Build history of the part. All positions in model axes, mm. A direction names the side the tool comes from. Give positions to 0.01 mm unless a question says otherwise; leave off trailing zeros. Write each loop counter-clockwise with the first axis right and the second up, starting at its lowest first coordinate (ties: lowest second). Pieces come first, ordered by that corner, then holes. Notation, with made-up numbers: (-7, 57) -> (19, 57) arc R5 ccw to (19, 64) -> close; hole circle Ø3 at (11, 8). An arc over 180 degrees is marked (long way). One line per question, with ' | ' between items. Start each with the question number.
(1) Tool access for faces 4 (the flat face through (-2.5, 0, -1)), 5 (the cylindrical face through (-1.43, 0.13, 0.45)), 6 (the flat face through (2.5, 0, -1)): list every direction of +Z, -Z, +X, -X, +Y, -Y with a clear straight run to the whole face (end or side of a thin tool).
(2) Pin check, flat tips, straight feed: P1, Ø0.6, axis at y = -2, z = -1, coming from the +X side; P2, Ø8, axis at x = 5, y = 5, coming from the -Z side; P3, Ø1, axis at y = 2.5, z = -1, coming from the -X side; P4, Ø7, axis at x = 6.5, y = 1.5, coming from the -Z side. Stop position of each tip, or through.
(3) Band-saw the part on C-C, the plane z = 2.5. Give the cut face in (x, y).
(4) Pull direction X, two halves, no side cores. Call faces 1 (the cylindrical face through (-2.215, -0.126, -2.699)), 2 (the flat face through (6, 0, 0)), 3 (the cylindrical face through (-4.737, 6.676, 1.521)): released by +X, released by -X, zero draft, split by the parting line, or undercut.
(5) Band-saw the part on A-A, the plane x = 0. Give the cut face in (y, z).
(6) Band-saw the part on D-D, the plane y = -3.5. Give the cut face in (x, z).
(7) Band-saw the part on B-B, the plane y = 6. Give the cut face in (x, z).
(8) Drill centre lines: probe 1 along Y at (x, z) = (-4, 1.95); probe 2 along Z at (x, y) = (0, -3.5); probe 3 along Z at (x, y) = (6.5, 2.25). Where is each one in solid material? Low to high. Write a range as from..to.
from build123d import *

# Parameters (mm, degrees)
SKETCH_1_W          = 18
SKETCH_1_H          = 18
EXTRUDE_1_DEPTH     = 3
SKETCH_4_R          = 1
CUT_EXTRUDE_1_DEPTH = 14.076696831
SKETCH_8_W          = 5
SKETCH_8_H          = 3
EXTRUDE_4_DEPTH     = 18
SKETCH_9_R          = 1.5
CUT_EXTRUDE_3_DEPTH = 21.346989949
FILLET_3_R          = 1


with BuildPart() as part:
    # 草图1 → 凸台-拉伸1 (new body)
    with BuildSketch(Plane.XY):
        Rectangle(SKETCH_1_W, SKETCH_1_H)
    extrude(amount=EXTRUDE_1_DEPTH)

    # 草图4 → 切除-拉伸1 (cut, through all)
    with BuildSketch(Plane.XY.offset(3)):
        with Locations((-4, -6)):
            Circle(SKETCH_4_R)
        with Locations((4, -6)):
            Circle(SKETCH_4_R)
        with Locations((4, 6)):
            Circle(SKETCH_4_R)
        with Locations((-4, 6)):
            Circle(SKETCH_4_R)
    extrude(amount=-CUT_EXTRUDE_1_DEPTH, mode=Mode.SUBTRACT)

    # 草图8 → 凸台-拉伸4 (add)
    with BuildSketch(Plane(origin=(0, 9, 0), x_dir=(1, 0, 0), z_dir=(0, 1, 0))):
        with Locations((0, 1.5)):
            Rectangle(SKETCH_8_W, SKETCH_8_H)
    extrude(amount=-EXTRUDE_4_DEPTH)

    # 草图9 → 切除-拉伸3 (cut, through all)
    with BuildSketch(Plane(origin=(0, 9, 0), x_dir=(1, 0, 0), z_dir=(0, 1, 0))):
        with Locations(Location((0, 0, 0), (0, 0, 180))):
            Circle(SKETCH_9_R)
    extrude(amount=-CUT_EXTRUDE_3_DEPTH, mode=Mode.SUBTRACT)

    # 圆角3
    fillet_3_edges = [part.edges().sort_by_distance(p)[0] for p in [
        (-2.5, 0, -3),
        (2.5, 0, -3),
    ]]
    fillet(fillet_3_edges, radius=FILLET_3_R)


solid = part.part
Results:
1) face 4: -Z, -X, +Y, -Y | face 5: +Y, -Y | face 6: -Z, +X, +Y, -Y
2) P1: stops at x = 2.5 | P2: stops at z = -3 | P3: stops at x = -2.5 | P4: stops at z = 0
3) outline: (-9, -9) -> (9, -9) -> (9, 9) -> (-9, 9) -> close; hole circle Ø2 at (-4, -6); hole circle Ø2 at (-4, 6); hole circle Ø2 at (4, -6); hole circle Ø2 at (4, 6)
4) face 1: released by -X | face 2: zero draft | face 3: undercut
5) outline: (-9, -3) -> (9, -3) -> (9, -1.5) -> (-9, -1.5) -> close; (-9, 1.5) -> (9, 1.5) -> (9, 3) -> (-9, 3) -> close
6) outline: (-9, 0) -> (-2.5, 0) -> (-2.5, -2) arc R1 ccw to (-1.5, -3) -> (1.5, -3) arc R1 ccw to (2.5, -2) -> (2.5, 0) -> (9, 0) -> (9, 3) -> (-9, 3) -> close; hole circle Ø3 at (0, 0)
7) outline: (-9, 0) -> (-5, 0) -> (-5, 3) -> (-9, 3) -> close; (-3, 0) -> (-2.5, 0) -> (-2.5, -2) arc R1 ccw to (-1.5, -3) -> (1.5, -3) arc R1 ccw to (2.5, -2) -> (2.5, 0) -> (3, 0) -> (3, 3) -> (-3, 3) -> close; (5, 0) -> (9, 0) -> (9, 3) -> (5, 3) -> close; hole circle Ø3 at (0, 0)
8) probe 1: y = -9..-7, -5..5, 7..9 | probe 2: z = -3..-1.5, 1.5..3 | probe 3: z = 0..3
